For this review, take the finished solid that the model builds, in its own axes (mm). A direction names the side the tool comes from. Round coordinates to 2 decimals unless told otherwise and drop trailing zeros. Order: outer loops, then holes, each group sorted by start corner. A loop starts at its lowest first (then second) coordinate and runs counter-clockwise, first axis right, second up. Notation, with made-up numbers: (46, -16.75) - (93, -16.75) arc R22 ccw to (93, 16.25) - close; hole circle Ø4 at (15.25, 0.5). An arc over 180 degrees is marked (long way). One line per question, with ' | ' between items.
Autodesk Inventor part; units mm, degrees
ref_plane "YZ Plane" through (0, 0, 0) normal (1, 0, 0) x (0, 1, 0)
ref_plane "XZ Plane" through (0, 0, 0) normal (0, 1, 0) x (-1, 0, 0)
ref_plane "XY Plane" through (0, 0, 0) normal (0, 0, 1) x (1, 0, 0)
sketch "Sketch1" plane through (0, 0, 0) normal (0, 1, 0) x (-1, 0, 0)
  line L0 (0, 0) -> (-25.4, 0)
  line L1 (-25.4, 0) -> (-25.4, -3.81)
  line L2 (-25.4, -3.81) -> (0, -3.81)
  line L3 (0, -3.81) -> (0, 0)
  line L4 (0, 0) -> (-3.81, 0)
  line L5 (-3.81, 0) -> (-3.81, -25.4)
  line L6 (-3.81, -25.4) -> (0, -25.4)
  line L7 (0, -25.4) -> (0, 0)
  point P0 (-3.81, -3.81)
  dimension "d0" = 25.4
  dimension "d1" = 3.81
  dimension "d2" = 3.81
  dimension "d3" = 25.4
extrude "Extrusion1" add sketch "Sketch1" along normal blind 12.7
sketch "Sketch2" plane through (0, 12.7, 0) normal (0, 1, 0) x (1, 0, 0)
  line L0 (3.81, 3.81) -> (3.81, 25.4)
  line L1 (25.4, 3.81) -> (3.81, 3.81)
  line L2 (3.81, 25.4) -> (25.4, 3.81)
  line L3 (0, 0) -> (25.4, 0)
  line L4 (25.4, 3.81) -> (25.4, 0)
  line L5 (0, 25.4) -> (0, 0)
  line L6 (25.4, 0) -> (0, 0)
  line L7 (0, 0) -> (0, 25.4)
  line L8 (0, 25.4) -> (3.81, 25.4)
extrude "Extrusion2" add sketch "Sketch2" along normal blind 6.35
sketch "Sketch3" plane through (0, 0, 0) normal (0, -1, 0) x (1, 0, 0)
  line L0 (3.81, -25.4) -> (0, -25.4)
  line L1 (0, -25.4) -> (3.81, -25.4)
  line L2 (25.4, -3.81) -> (3.81, -25.4)
  line L3 (3.81, -25.4) -> (25.4, -3.81)
  line L4 (25.4, 0) -> (25.4, -3.81)
  line L5 (25.4, -3.81) -> (25.4, 0)
  line L6 (0, 0) -> (25.4, 0)
  line L7 (25.4, 0) -> (0, 0)
  line L8 (0, 0) -> (0, -25.4)
extrude "Extrusion3" add sketch "Sketch3" along normal blind 6.35
sketch "Sketch4" plane through (0, 12.7, 0) normal (0, -1, 0) x (1, 0, 0)
  line L0 (3.81, -25.4) -> (25.4, -3.81)
  line L1 (15.875, -13.335) -> (12.2829, -9.7429)
  line L2 (12.2829, -9.7429) -> (3.81, -18.2158)
  line L3 (3.81, -3.81) -> (3.81, -25.4)
  line L4 (25.4, -3.81) -> (3.81, -3.81)
  line L5 (3.81, -18.2158) -> (3.81, -3.81)
  line L6 (3.81, -3.81) -> (18.2158, -3.81)
  line L7 (12.2829, -9.7429) -> (18.2158, -3.81)
  dimension "d10" = 5.08
extrude "Extrusion4" cut sketch "Sketch4" against normal mid plane 50.8 contours L3 L4 L7 L2
sketch "Sketch5" plane through (3.81, -6.35, -3.81) normal (1, 0, 0) x (0, 0, -1)
  line L0 (0, 6.35) -> (0, 19.05)
  line L1 (0, 12.7) -> (21.59, 12.7)
  line L2 (21.59, 6.35) -> (21.59, 19.05)
  circle A0 centre (6.35, 12.7) radius 3.429
  circle A1 centre (15.6845, 16.129) radius 2
  circle A2 centre (15.6845, 9.525) radius 2
  line L3 (9.779, 12.7) -> (21.59, 12.7)
  line L4 (15.6845, 12.7) -> (15.6845, 6.35)
  line L5 (14.4058, 6.35) -> (21.59, 6.35)
  line L6 (15.6845, 12.7) -> (15.6845, 19.05)
  line L7 (14.4058, 19.05) -> (21.59, 19.05)
  circle A3 centre (6.35, 12.9362) radius 6.35
  dimension "d13" = 6.858
  dimension "d16" = 4
  dimension "d17" = 4
  dimension "d18" = 12.7
extrude "Extrusion5" cut sketch "Sketch5" against normal blind 12.7 contours A0 L1 | L1 A0 | L4 A2 | A2 L4 | L6 A1 | A1 L6
sketch "Sketch6" plane through (3.81, -6.35, -3.81) normal (0, 0, -1) x (-1, 0, 0)
  line L0 (0, 6.35) -> (0, 19.05)
  line L1 (0, 12.7) -> (21.59, 12.7)
  line L2 (21.59, 6.35) -> (21.59, 19.05)
  circle A0 centre (6.35, 12.7) radius 3.429
  circle A1 centre (15.6845, 16.129) radius 2
  circle A2 centre (15.6845, 9.525) radius 2
  line L3 (9.779, 12.7) -> (21.59, 12.7)
  line L4 (15.6845, 12.7) -> (15.6845, 6.35)
  line L5 (14.4058, 6.35) -> (21.59, 6.35)
  line L6 (15.6845, 12.7) -> (15.6845, 19.05)
  line L7 (14.4058, 19.05) -> (21.59, 19.05)
  circle A3 centre (6.35, 12.9362) radius 6.35
  line L8 (-15.6845, 12.7) -> (-15.6845, 6.35)
  circle A4 centre (-15.6845, 9.525) radius 2
  line L9 (-15.6845, 12.7) -> (-15.6845, 19.05)
  line L10 (-9.779, 12.7) -> (-21.59, 12.7)
  circle A5 centre (-15.6845, 16.129) radius 2
  line L11 (-14.4058, 6.35) -> (-21.59, 6.35)
  line L12 (-21.59, 6.35) -> (-21.59, 19.05)
  line L13 (-14.4058, 19.05) -> (-21.59, 19.05)
  line L14 (0, 12.7) -> (-21.59, 12.7)
  circle A6 centre (-6.35, 12.7) radius 3.429
  circle A7 centre (-6.35, 12.9362) radius 6.35
  dimension "d19" = 6.858
  dimension "d20" = 4
  dimension "d21" = 4
  dimension "d22" = 12.7
extrude "Extrusion6" cut sketch "Sketch6" against normal blind 12.7 contours A6 L14 | L14 A6 | A4 L8 | L8 A4 | A5 L9 | L9 A5
sketch "Sketch7" plane through (0, -6.35, 0) normal (0, -1, 0) x (1, 0, 0)
  line L0 (25.4, 0) -> (0, 0)
  line L1 (0, 0) -> (25.4, 0)
  line L2 (25.4, 0) -> (25.4, -25.4)
  line L3 (25.4, -25.4) -> (0, -25.4)
  line L4 (0, -25.4) -> (0, 0)
  dimension "d25" = 25.4
  dimension "d26" = 25.4
extrude "Extrusion7" add sketch "Sketch7" against normal blind 2.54
sketch "Sketch8" plane through (0, -3.81, 0) normal (0, 1, 0) x (1, 0, 0)
  circle A0 centre (10.16, 10.16) radius 6.35
  circle A1 centre (10.16, 10.16) radius 3.175
  line L0 (18.2158, 3.81) -> (3.81, 3.81)
  line L1 (3.81, 3.81) -> (3.81, 18.2158)
  dimension "d29" = 12.7
  dimension "d30" = 6.35
extrude "Extrusion8" cut sketch "Sketch8" against normal mid plane 10.16 contours A1
extrude "Extrusion9" cut sketch "Sketch8" along normal blind 10.16 contours A0
equation "\"d2\" = d1"
properties part number "panel connector" material "PC/ABS Plastic"
(1) We need section C-C on x = 7.75. State the section outline as (y, z) points, plus the area to 3 significant figures.
Output values:
outline: (-6.35, -25.4) - (-3.81, -25.4) - (-3.81, -21.46) - (0, -21.46) - (0, -16.03) - (-3.81, -16.03) - (-3.81, -12.23) - (-6.35, -12.23) - close; (-6.35, -8.09) - (-3.81, -8.09) - (-3.81, -3.81) - (3.91, -3.81) - (3.91, 0) - (-6.35, 0) - close; (8.79, -3.81) - (19.05, -3.81) - (19.05, 0) - (8.79, 0) - close; (12.7, -21.46) - (19.05, -21.46) - (19.05, -14.28) - (12.7, -14.28) - close | area: 189 mm^2
(2) We need section B-B on y = 6.35. State the section outline as (x, z) points, plus the area to 3 significant figures.
Output values:
outline: (0, -25.4) - (3.81, -25.4) - (3.81, -13.59) - (0, -13.59) - close; (0, -6.73) - (3.81, -6.73) - (3.81, -3.81) - (6.73, -3.81) - (6.73, 0) - (0, 0) - close; (13.59, -3.81) - (25.4, -3.81) - (25.4, 0) - (13.59, 0) - close | area: 127 mm^2
(3) Insertion check: pin 1 (8 mm diameter, centred on x = 11.5, y = 2, fed in from -Z); pin 2 (11 mm diameter, centred on y = 6.35, z = -10.16, fed in from +X); pin 3 (8 mm diameter, centred on x = 10.16, y = 6.35, fed in from -Z); pin 4 (3.5 mm diameter, centred on y = 9.78, z = -19.49, fed in from -X). Each pin has a flat end and moves straight along its axis. Give the tip position at first contact, or say it passes through.
Output values:
pin 1: z = -21.17 | pin 2: x = 3.81 | pin 3: z = -3.81 | pin 4: through
(4) Mouldability with a two-part tool opening along Z and no side actions: class faces 6 (the flat face through (8.96, -1.88, -20.25)), 7 (the cylindrical face through (1.93, 4.86, -20.57)), 8 (the flat face through (0, 9, -13)), 9 (the flat face through (13, 9, 0)) as released by +Z, released by -Z, zero draft, split by the parting line, or undercut.
Output values:
face 6: released by -Z | face 7: undercut | face 8: zero draft | face 9: released by +Z
(5) We need section A-A on z = -19.5. State the section outline as (x, y) points (3 decimals).
Output values:
outline: (0, -6.35) - (25.4, -6.35) - (25.4, -3.81) - (9.71, -3.81) - (9.71, 0) - (3.81, 0) - (3.81, 1.175) - (0, 1.175) - close; (0, 5.175) - (3.81, 5.175) - (3.81, 7.779) - (0, 7.779) - close; (0, 11.779) - (3.81, 11.779) - (3.81, 12.7) - (9.71, 12.7) - (9.71, 19.05) - (0, 19.05) - close
(6) We need section D-D on x = 22.5. State the section outline as (y, z) points, plus the area to 3 significant figures.
Output values:
outline: (-6.35, -25.4) - (-3.81, -25.4) - (-3.81, -6.71) - (0, -6.71) - (0, -3.81) - (12.7, -3.81) - (12.7, -6.71) - (19.05, -6.71) - (19.05, 0) - (-6.35, 0) - close | area: 181 mm^2
(7) For faces 1 (the flat face through (11.114, 15.831, -10.912)), 2 (the cylindrical face through (16.506, -1.932, -10.371)), 3 (the flat face through (13, 12.7, -13)), 4 (the flat face through (14.45, 15.83, -14.76)), 5 (the cylindrical face through (21.493, 3.263, -1.932)), list the 3-axis set-ups (+Z, -Z, +X, -X, +Y, -Y) from which the entire face can be reached by the end or side of a thin tool; tool diameter is ignored.
Output values:
face 1: +Y | face 2: none | face 3: -Z, +X | face 4: -Z, +X, +Y | face 5: +Z, -Z
(8) For probe 1 along Y at (x, z) = (10.16, -2.05); probe 2 along Y at (x, z) = (9, -14.5); probe 3 along Z at (x, y) = (10.16, -5.6) (3 decimals), list the stretches that pass through material, from the lowest coordinate up. Write a range as [from, to].
Output values:
probe 1: [-6.35, 2.92], [9.78, 19.05] | probe 2: [-6.35, -3.81], [12.7, 19.05] | probe 3: [-25.4, -13.335], [-6.985, 0]
